```python
from build123d import *

# Parameters (mm, degrees)
SKETCH_1_W                   = 38
SKETCH_1_H                   = 45
EXTRUDE_1_DEPTH              = 6
SKETCH_2_R                   = 12
SKETCH_2_R_2                 = 1.5
CUT_EXTRUDE_1_DEPTH          = 31.054117854
CUT_EXTRUDE_2_DEPTH          = 2
FILLET_2_R                   = 1
FILLET_3_R                   = 8
FILLET_4_R                   = 2
SKETCH_4_W                   = 10
SKETCH_4_H                   = 3
EXTRUDE_2_DEPTH              = 6
CHAMFER_1_SIZE               = 0.5
HOLE_WIZARD_M3_1_D           = 2.5
HOLE_WIZARD_M3_1_DEPTH       = 7.5
HOLE_WIZARD_M3_1_CSINK_D     = 3.05
HOLE_WIZARD_M3_1_CSINK_ANGLE = 90
HOLE_WIZARD_M3_1_TIP         = 0.751075774


with BuildPart() as part:
    # 草图1 → 凸台-拉伸1 (new body)
    with BuildSketch(Plane(origin=(0, 0, 0), x_dir=(0, 0, -1), z_dir=(1, 0, 0))):
        Rectangle(SKETCH_1_W, SKETCH_1_H)
    extrude(amount=EXTRUDE_1_DEPTH)

    # 草图2 → 切除-拉伸1 (cut, through all)
    with BuildSketch(Plane.ZY):
        with Locations((0, -7.5)):
            Circle(SKETCH_2_R)
        with Locations((15, -7.5)):
            Circle(SKETCH_2_R_2)
        with Locations(Location((-15, -7.5, 0), (0, 0, 180))):
            Circle(SKETCH_2_R_2)
    extrude(amount=-CUT_EXTRUDE_1_DEPTH, mode=Mode.SUBTRACT)

    # 草图3 → 切除-拉伸2 (cut)
    with BuildSketch(Plane.ZY):
        with BuildLine():
            Line((19.25, -7.5), (19.25, -22.5))
            Line((19.25, -22.5), (-19.25, -22.5))
            Line((-19.25, -22.5), (-19.25, -7.5))
            ThreePointArc((-19.25, -7.5), (0, 11.75), (19.25, -7.5))
        make_face()
    extrude(amount=-CUT_EXTRUDE_2_DEPTH, mode=Mode.SUBTRACT)

    # 圆角2
    fillet_2_edges = [part.edges().sort_by_distance(p)[0] for p in [
        (1, -4.407670781, -19),
        (1, -4.407670781, 19),
    ]]
    fillet(fillet_2_edges, radius=FILLET_2_R)

    # 圆角3
    fillet_3_edges = [part.edges().sort_by_distance(p)[0] for p in [
        (4, -22.5, -19),
        (4, -22.5, 19),
    ]]
    fillet(fillet_3_edges, radius=FILLET_3_R)

    # 圆角4
    fillet_4_edges = [part.edges().sort_by_distance(p)[0] for p in [
        (3, 22.5, 19),
        (3, 22.5, -19),
    ]]
    fillet(fillet_4_edges, radius=FILLET_4_R)

    # 草图4 → 凸台-拉伸2 (add)
    with BuildSketch(Plane.ZY):
        with Locations((0, 24)):
            Rectangle(SKETCH_4_W, SKETCH_4_H)
    extrude(amount=-EXTRUDE_2_DEPTH)

    # 倒角1
    chamfer_1_edges = [part.edges().sort_by_distance(p)[0] for p in [
        (3, 25.5, 5),
        (3, 25.5, -5),
    ]]
    chamfer(chamfer_1_edges, length=CHAMFER_1_SIZE)

    # M3 螺纹孔1
    with Locations(Plane(origin=(3, 22.5, -11), x_dir=(0, 0, 1), z_dir=(0, 1, 0))):
        with Locations((0, 0), (22, 0)):
            CounterSinkHole(HOLE_WIZARD_M3_1_D / 2, HOLE_WIZARD_M3_1_CSINK_D / 2, depth=HOLE_WIZARD_M3_1_DEPTH, counter_sink_angle=HOLE_WIZARD_M3_1_CSINK_ANGLE)
            with Locations((0, 0, -(HOLE_WIZARD_M3_1_DEPTH + HOLE_WIZARD_M3_1_TIP / 2))):  # 118° drill point
                Cone(0, HOLE_WIZARD_M3_1_D / 2, HOLE_WIZARD_M3_1_TIP, mode=Mode.SUBTRACT)


solid = part.part
```
Geometry: final body of the model. Coordinates: model frame, mm. A direction names the side the tool comes from. Round coordinates to 2 decimals unless told otherwise and drop trailing zeros. Order: outer loops, then holes, each group sorted by start corner. A loop starts at its lowest first (then second) coordinate and runs counter-clockwise, first axis right, second up. Notation, with made-up numbers: (9.5, 57.5) -> (58.5, 57.5) arc R21 cw to (58.5, 86.5) -> close; hole circle Ø6 at (54.5, 12.5). An arc over 180 degrees is marked (long way). Write each question's results on one line, items separated by ' | '.
Q1. Pin query (flat end, axial travel): pin 1 Ø3 at (x, y) = (3, 23) entering from -Z; pin 2 Ø5 at (y, z) = (8, 4) entering from -X; pin 3 Ø2 at (x, y) = (1.5, 24) entering from +Z. Return the tip coordinate at first contact, or that it passes through.
Response values:
pin 1: z = -18.73 | pin 2: x = 2 | pin 3: z = 5
Q2. Section query D-D (y = -16.5). Output: boundary loops of the cut face in (x, z), and give its area (3 significant figures).
Response values:
outline: (2, -18.75) -> (6, -18.75) -> (6, -7.94) -> (2, -7.94) -> close; (2, 7.94) -> (6, 7.94) -> (6, 18.75) -> (2, 18.75) -> close | area: 86.5 mm²
Q3. Ray query, line 1 along Z through (x, y) = (3, 17); line 2 along X through (y, z) = (17.75, 11); line 3 along X through (y, z) = (-2, 15). Return the intervals inside material, ascending.
Response values:
line 1: -19 to -12.25, -9.75 to 9.75, 12.25 to 19 | line 2: 0 to 1.75, 4.25 to 6 | line 3: 2 to 6
Q4. Section query C-C (x = 0.6). Output: boundary loops of the cut face in (y, z), and give its area (3 significant figures).
Response values:
outline: (1.32, -17.11) arc R1 ccw to (1.78, -19) -> (20.5, -19) arc R2 ccw to (22.5, -17) -> (22.5, -5) -> (25, -5) -> (25.5, -4.5) -> (25.5, 4.5) -> (25, 5) -> (22.5, 5) -> (22.5, 17) arc R2 ccw to (20.5, 19) -> (1.78, 19) arc R1 ccw to (1.32, 17.11) arc R19.25 cw to start | area: 579 mm²
Q5. Section query A-A (y = -7.5). Output: boundary loops of the cut face in (x, z), and give its area (3 significant figures).
Response values:
outline: (2, -19) -> (6, -19) -> (6, -16.5) -> (2, -16.5) -> close; (2, -13.5) -> (6, -13.5) -> (6, -12) -> (2, -12) -> close; (2, 12) -> (6, 12) -> (6, 13.5) -> (2, 13.5) -> close; (2, 16.5) -> (6, 16.5) -> (6, 19) -> (2, 19) -> close | area: 32.0 mm²
Q6. Access query for faces 1 (the face through (4, 3, -19)), 2 (the face through (0.99, 0.8, -18.22)), 3 (the face through (3.97, -6.97, -11.99)), 4 (the face through (1.6, 22.5, 12.4)), 5 (the face through (1.6, 22.5, -9.6)). Directions: +Z, -Z, +X, -X, +Y, -Y. A direction counts if a zero-diameter tool reaches every point of the face in a straight line with its end or side. Return the directions, or none.
Response values:
face 1: -Z, +X, -X, +Y, -Y | face 2: -X, -Y | face 3: +X, -X | face 4: +Z, +X, -X, +Y | face 5: -Z, +X, -X, +Y
Q7. Section query B-B (z = 15). Output: boundary loops of the cut face in (x, y).
Response values:
outline: (0, 4.56) -> (2, 4.56) -> (2, -6) -> (6, -6) -> (6, 22.5) -> (0, 22.5) -> close; (2, -21.43) -> (6, -21.43) -> (6, -9) -> (2, -9) -> close
Q8. Pull-direction query (X, two-part tool) for faces 6 (the face through (3.05, 18.56, 12.25)), 7 (the face through (4, 3, 19)), 8 (the face through (0, 16, 0)); classes: released by +X, released by -X, zero draft, split by the parting line, or undercut.
Response values:
face 6: undercut | face 7: zero draft | face 8: released by -X
